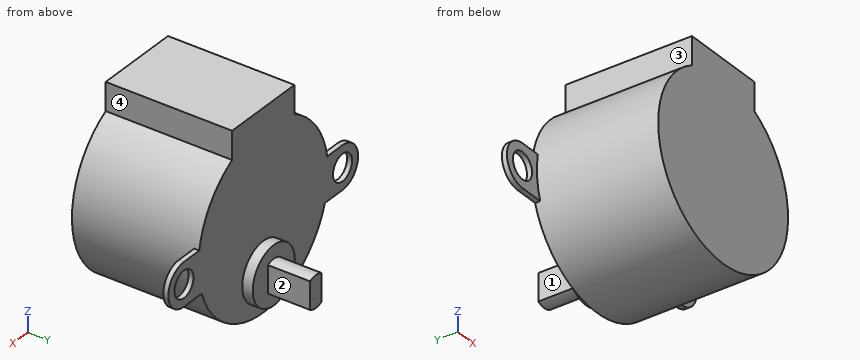
from build123d import *

# Parameters (mm, degrees)
BOSS_EXTRUDE1_DEPTH = 19.05
BOSS_EXTRUDE2_START = -0.762
SKETCH3_R           = 1.984375
BOSS_EXTRUDE2_DEPTH = 0.762
SKETCH5_R           = 4.365625
BOSS_EXTRUDE3_DEPTH = 1.5875
BOSS_EXTRUDE4_DEPTH = 6.35


with BuildPart() as part:
    # Sketch2 → Boss-Extrude1 (new body)
    with BuildSketch(Plane(origin=(0, 0, 0), x_dir=(1, 0, 0), z_dir=(0, 1, 0))):
        with BuildLine():
            Line((6.477, -16.053488894), (6.477, -11.83764166))
            ThreePointArc((6.477, -11.83764166), (0, 13.49375), (-6.477, -11.83764166))
            Line((-6.477, -11.83764166), (-6.477, -16.053488894))
            Line((-6.477, -16.053488894), (6.477, -16.053488894))
        make_face()
    extrude(amount=BOSS_EXTRUDE1_DEPTH)

    # Sketch3 → Boss-Extrude2 (add)
    # profile 1 of 2: a face of its own
    with BuildSketch(Plane(origin=(0, 19.05, 0), x_dir=(1, 0, 0), z_dir=(0, 1, 0)).offset(BOSS_EXTRUDE2_START)):
        with BuildLine():
            ThreePointArc((-16.479121392, 4.22275), (-19.717621392, 0.98425), (-16.479121392, -2.25425))
            Line((-16.479121392, -2.25425), (-13.304121392, -2.25425))
            ThreePointArc((-13.304121392, -2.25425), (-13.455592652, 1.014058895), (-12.815992802, 4.22275))
            Line((-12.815992802, 4.22275), (-16.479121392, 4.22275))
        make_face()
        with Locations(Location((-16.479121392, 0.98425, 0), (0, 0, 270))):
            Circle(SKETCH3_R, mode=Mode.SUBTRACT)
    # profile 2 of 2: a face of its own
    with BuildSketch(Plane(origin=(0, 19.05, 0), x_dir=(1, 0, 0), z_dir=(0, 1, 0)).offset(BOSS_EXTRUDE2_START)):
        with BuildLine():
            Line((16.479121392, 4.22275), (12.815992802, 4.22275))
            ThreePointArc((12.815992802, 4.22275), (13.455592652, 1.014058895), (13.304121392, -2.25425))
            Line((13.304121392, -2.25425), (16.479121392, -2.25425))
            ThreePointArc((16.479121392, -2.25425), (19.717621392, 0.98425), (16.479121392, 4.22275))
        make_face()
        with Locations(Location((16.479121392, 0.98425, 0), (0, 0, 270))):
            Circle(SKETCH3_R, mode=Mode.SUBTRACT)
    extrude(amount=BOSS_EXTRUDE2_DEPTH)

    # Sketch5 → Boss-Extrude3 (add)
    with BuildSketch(Plane(origin=(0, 19.05, 0), x_dir=(1, 0, 0), z_dir=(0, 1, 0))):
        with Locations(Location((0, 7.501133667, 0), (0, 0, 270))):
            Circle(SKETCH5_R)
    extrude(amount=BOSS_EXTRUDE3_DEPTH)

    # Sketch6 → Boss-Extrude4 (add)
    with BuildSketch(Plane(origin=(0, 20.6375, 0), x_dir=(1, 0, 0), z_dir=(0, 1, 0))):
        with BuildLine():
            ThreePointArc((1.190625, 9.56335666), (0, 9.882383667), (-1.190625, 9.56335666))
            Line((-1.190625, 9.56335666), (-1.190625, 5.438910675))
            ThreePointArc((-1.190625, 5.438910675), (0, 5.119883667), (1.190625, 5.438910675))
            Line((1.190625, 5.438910675), (1.190625, 9.56335666))
        make_face()
    extrude(amount=BOSS_EXTRUDE4_DEPTH)


solid = part.part
Check sheet for the modelled part. Datum: model origin and axes. Units: mm. Face numbers are marked on the shaded views. A direction names the side the tool comes from. Give positions to 0.01 mm unless a question says otherwise; leave off trailing zeros. Write each loop counter-clockwise with the first axis right and the second up, starting at its lowest first coordinate (ties: lowest second). Pieces come first, ordered by that corner, then holes. Notation, with made-up numbers: M 49,-34.5 L 90,-34.5 A26 cw 90,1.5 Z; hole C -7.5,-2.5 d2. An arc over 180 degrees is marked long. Use one line per item in the form item = value.
(1) Section check D-D on y = 22. Record the boundary of the cut face in (x, z).
Answer block:
outline = M -1.19,-9.56 A2.38 ccw 1.19,-9.56 L 1.19,-5.44 A2.38 ccw -1.19,-5.44 Z
(2) Material ranges on line 1 along Y through (x, z) = (12, -2.25); line 2 along Y through (x, z) = (-15, -3); line 3 along X through (y, z) = (11, 14.25), recorded low to high.
Answer block:
line_1 = 0 to 19.05
line_2 = 18.29 to 19.05
line_3 = -6.48 to 6.48
(3) Section check B-B on x = -15. Record the boundary of the cut face in (y, z), plus the area to 3 significant figures.
Answer block:
outline = M 18.29,-4.22 L 19.05,-4.22 L 19.05,-2.31 L 18.29,-2.31 Z; M 18.29,0.34 L 19.05,0.34 L 19.05,2.25 L 18.29,2.25 Z
area = 2.92 mm2
(4) Section check A-A on z = 0.5. Record the boundary of the cut face in (x, y).
Answer block:
outline = M -19.36,18.29 L -17.8,18.29 L -17.8,19.05 L -19.36,19.05 Z; M -15.16,18.29 L -13.48,18.29 L -13.48,0 L 13.48,0 L 13.48,18.29 L 15.16,18.29 L 15.16,19.05 L -15.16,19.05 Z; M 17.8,18.29 L 19.36,18.29 L 19.36,19.05 L 17.8,19.05 Z
(5) Depth check by flat-ended pin: P1, Ø0.8, axis at x = -14, y = 18.5, coming from the -Z side; P2, Ø1.5, axis at x = 9, z = 2.5, coming from the +Y side; P3, Ø1.2, axis at y = 23, z = -7, coming from the -X side. Enter the tip coordinate at first touch or a pass-through.
Answer block:
P1 = -4.22
P2 = 19.05
P3 = -1.19
(6) Tool access check on the marked faces 1, 2, 3 and 4. Record the directions out of +Z, -Z, +X, -X, +Y, -Y that give a thin tool (end or side, any length) a straight path to the whole face; none if there is none.
Answer block:
face_1 = +Z, -Z, -X, +Y
face_2 = +Z, -Z, +X, +Y
face_3 = +Z, -X, +Y, -Y
face_4 = +Z, +X, +Y, -Y
(7) Section check C-C on z = -9. Record the boundary of the cut face in (x, y).
Answer block:
outline = M -10.05,0 L 10.05,0 L 10.05,19.05 L 4.1,19.05 L 4.1,20.64 L 1.19,20.64 L 1.19,26.99 L -1.19,26.99 L -1.19,20.64 L -4.1,20.64 L -4.1,19.05 L -10.05,19.05 Z
